Autodesk Fusion 360 part; units mm, degrees
sketch "Skizze1" plane through (0, 0, 0) normal (0, 0, 1) x (1, 0, 0)
  circle A0 centre (0, 0) radius 41
  circle A1 centre (24.5, 24.5) radius 2.25
  circle A2 centre (24.5, -24.5) radius 2.25
  circle A3 centre (-24.5, -24.5) radius 2.25
  circle A4 centre (-24.5, 24.5) radius 2.25
  dimension "d1" = 82
  dimension "d4" = 49
  dimension "d5" = 49
  dimension "d6" = 4.5
  dimension "d7" = 4.5
  dimension "d8" = 4.5
  dimension "d9" = 4.5
extrude "Extrusion1" add sketch "Skizze1" along normal blind 5
chamfer "Fase1" distance 1 angle 45 1 edges at (-38.2254, -14.8262, 5)
sketch "Skizze2" plane through (0, 0, 5) normal (0, 0, 1) x (-1, 0, 0)
  circle A0 centre (-24.5, -24.5) radius 2.25
  circle A1 centre (24.5, 24.5) radius 2.25
  circle A2 centre (-24.5, 24.5) radius 2.25
  circle A3 centre (24.5, -24.5) radius 2.25
  circle A4 centre (0, 0) radius 40
hole "Bohrung1" at (0, 0, 5) direction (0, 0, -1) diameter 8 depth 5 tip angle 118 countersink diameter 16 countersink angle 90
Design review of the part built by this model. Coordinates are the model's own, in mm. Coordinates: 2 decimals unless noted, no trailing zeros. Loops run counter-clockwise (first coordinate to the right, second up) from the corner with the lowest first, then second, coordinate; pieces in that order, holes last. Notation, with made-up numbers: (61.25, -33) -> (112.25, -33) arc R10 cw to (112.25, -27) -> close; hole circle Ø1 at (35, 76). An arc over 180 degrees is marked (long way). Use a Markdown table: item, result. Add a question column.
Item 1: We need section C-C, the plane z = 2.25. Write out the cut boundary in (x, y).
Item 2: Clearance check with a flat-ended pin moving along its axis: P1, Ø1, axis at x = -24.5, z = 3.5, coming from the +Y side. State where the tip first meets the part, or that it passes through.
Item 3: Wall thickness on L1, parallel to X at y = 23, z = 2.35; L2, parallel to Y at x = 24.5, z = 1.7; L3, parallel to Y at x = 26, z = 3.95: over which ranges is each line inside the solid? List them lowest first. Write a range as from..to.
Item 4: We need section A-A, the plane x = 0. Write out the cut boundary in (y, z).
Item 5: We need section D-D, the plane x = 24.5. Count the separate pieces of the cut face and the enclosed holes in it, and give its area (3 significant figures).
Item 6: The part is to be moulded in two halves that separate along X. For faces 1 (the cylindrical face through (-9, 40, 2)), 2 (the cylindrical face through (25.538, 26.496, 2.465)), 3 (the flat face through (-1, -9, 0)), 4 (the cylindrical face through (-23.462, -22.504, 2.465)), say which applies: +X half, -X half, draft (parallel to the pull), parting line (faces both ways), or undercut.
Numbers:
| question | item | result |
|---|---|---|
| 1 | outline | circle Ø82 at (0, 0); hole circle Ø4.5 at (-24.5, -24.5); hole circle Ø4.5 at (-24.5, 24.5); hole circle Ø10.5 at (0, 0); hole circle Ø4.5 at (24.5, -24.5); hole circle Ø4.5 at (24.5, 24.5) |
| 2 | P1 | stops at y = 33.24 |
| 3 | L1 | x = -33.94..-26.18, -22.82..22.82, 26.18..33.94 |
| 3 | L2 | y = -32.87..-26.75, -22.25..22.25, 26.75..32.87 |
| 3 | L3 | y = -31.7..-26.18, -22.82..22.82, 26.18..31.7 |
| 4 | outline | (-41, 0) -> (-4, 0) -> (-4, 1) -> (-8, 5) -> (-40, 5) -> (-41, 4) -> close; (4, 0) -> (41, 0) -> (41, 4) -> (40, 5) -> (8, 5) -> (4, 1) -> close |
| 5 | separate pieces | 3 |
| 5 | enclosed holes | 0 |
| 5 | area | 282 mm^2 |
| 6 | face 1 | parting line |
| 6 | face 2 | undercut |
| 6 | face 3 | draft |
| 6 | face 4 | undercut |
